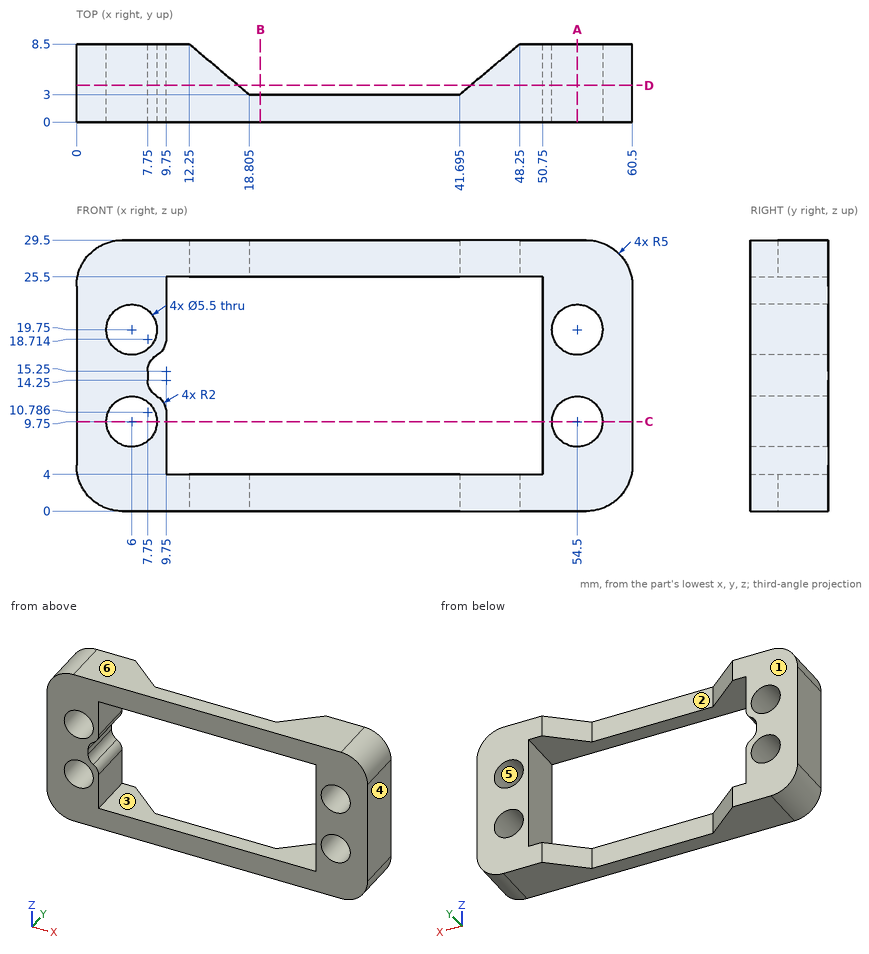
Verification items for this drawing (mm, ordinates from the low corner). A direction names the side the tool comes from. Round coordinates to 2 decimals unless told otherwise and drop trailing zeros. Loops run counter-clockwise (first coordinate to the right, second up) from the corner with the lowest first, then second, coordinate; pieces in that order, holes last. Notation, with made-up numbers: (0.5, 5) -> (32.5, 5) arc R26 cw to (32.5, 32) -> close; hole circle Ø10 at (10, 78). An arc over 180 degrees is marked (long way). Write item = value, one per line. Start each with the question number.
1) Gauge pin test, flat ends, axial feed: pin 1 Ø5 at (x, z) = (6, 9.75) entering from +Y; pin 2 Ø2 at (x, z) = (34.5, 2.5) entering from +Y. Record the tip position at first contact, or that the pin passes through.
2) Sectioned sample at C-C, the plane z = 9.75. Record the cut outline in (x, y).
3) Release check for a two-part mould opening along X. For the marked faces 4, 5 and 6 record: released by +X, released by -X, zero draft, split by the parting line, or undercut.
4) Set-up check for the marked faces 1, 2 and 3: record each of +Z, -Z, +X, -X, +Y, -Y from which the full face is reachable in a straight line by a thin tool's end or side.
5) Sectioned sample at A-A, the plane x = 54.5. Record the cut outline in (y, z), plus the area to 3 significant figures.
6) Sectioned sample at D-D, the plane y = 4. State how many separate pieces and enclosed holes the cut face has.
7) Thickness scan on probe 1 along Z at (x, y) = (54.5, 2); probe 2 along Z at (x, y) = (18.5, 3); probe 3 along X at (y, z) = (6.75, 4.75). Record the ranges inside material, lowest first.
8) Sectioned sample at B-B, the plane x = 20. Record the cut outline in (y, z).
Results are:
q1.pin_1 = through
q1.pin_2 = 3
q2.outline = (0, 0) -> (3.25, 0) -> (3.25, 8.5) -> (0, 8.5) -> close; (8.75, 0) -> (9.75, 0) -> (9.75, 8.5) -> (8.75, 8.5) -> close; (50.75, 0) -> (51.75, 0) -> (51.75, 8.5) -> (50.75, 8.5) -> close; (57.25, 0) -> (60.5, 0) -> (60.5, 8.5) -> (57.25, 8.5) -> close
q3.face_4 = released by +X
q3.face_5 = undercut
q3.face_6 = zero draft
q4.face_1 = +Z, -Z, +X, -X, +Y
q4.face_2 = +Z, -Z, +Y
q4.face_3 = +Y, -Y
q5.outline = (0, 0) -> (8.5, 0) -> (8.5, 7) -> (0, 7) -> close; (0, 12.5) -> (8.5, 12.5) -> (8.5, 17) -> (0, 17) -> close; (0, 22.5) -> (8.5, 22.5) -> (8.5, 29.5) -> (0, 29.5) -> close
q5.area = 157 mm^2
q6.separate_pieces = 2
q6.enclosed_holes = 4
q7.probe_1 = 0 to 7, 12.5 to 17, 22.5 to 29.5
q7.probe_2 = 0 to 4, 25.5 to 29.5
q7.probe_3 = 0.01 to 9.75, 50.75 to 60.49
q8.outline = (0, 0) -> (3, 0) -> (3, 4) -> (0, 4) -> close; (0, 25.5) -> (3, 25.5) -> (3, 29.5) -> (0, 29.5) -> close
